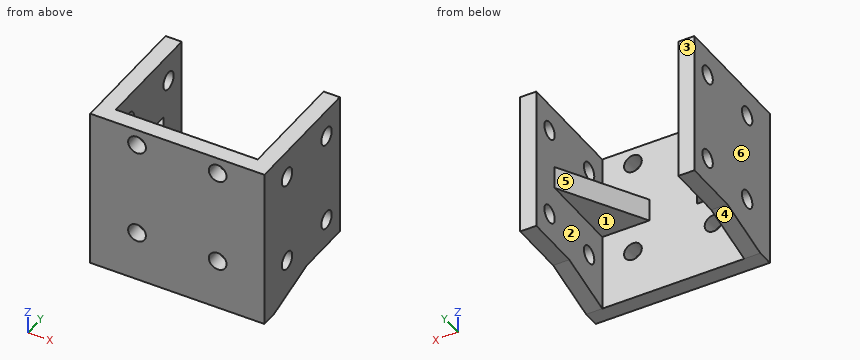
from build123d import *

# Parameters (mm, degrees)
SKETCH1_W               = 54
SKETCH1_H               = 55
BOSS_EXTRUDE1_DEPTH     = 5
SKETCH6_W               = 5
SKETCH6_H               = 45
BOSS_EXTRUDE3_DEPTH     = 35
SKETCH7_R               = 2.75
CUT_EXTRUDE2_DEPTH      = 69.972820734
RIB1_REACH              = 74.61
SKETCH8_WALL_W          = 165.420796688
SKETCH8_WALL_H          = 5
MIRROR2_COPY_1_REACH    = 74.61
MIRROR2_COPY_1_SKETCH_W = 165.420796688
MIRROR2_COPY_1_SKETCH_H = 5
RIB4_REACH              = 57.545
SKETCH9_WALL_W          = 142.246242154
SKETCH9_WALL_H          = 7
SKETCH10_R              = 2.75
CUT_EXTRUDE3_DEPTH      = 53.060061468
SKETCH11_W              = 54
SKETCH11_H              = 5
CUT_EXTRUDE4_DEPTH      = 40


with BuildPart() as part:
    # Sketch1 → Boss-Extrude1 (new body)
    with BuildSketch(Plane(origin=(0, 0, 0), x_dir=(1, 0, 0), z_dir=(0, 1, 0))):
        Rectangle(SKETCH1_W, SKETCH1_H)
    extrude(amount=BOSS_EXTRUDE1_DEPTH)

    # Sketch6 → Boss-Extrude3 (add)
    with BuildSketch(Plane(origin=(0, 5, 0), x_dir=(1, 0, 0), z_dir=(0, 1, 0))):
        with Locations((-24.5, 0)):
            Rectangle(SKETCH6_W, SKETCH6_H)
    boss_extrude3 = extrude(amount=BOSS_EXTRUDE3_DEPTH)

    # Sketch7 → Cut-Extrude2 (cut, through all)
    with BuildSketch(Plane(origin=(-22, 0, 0), x_dir=(0, 0, -1), z_dir=(1, 0, 0))):
        with Locations((-14, 33)):
            Circle(SKETCH7_R)
        with Locations((14, 33)):
            Circle(SKETCH7_R)
        with Locations((14, 12)):
            Circle(SKETCH7_R)
        with Locations((-14, 12)):
            Circle(SKETCH7_R)
    cut_extrude2 = extrude(amount=-CUT_EXTRUDE2_DEPTH, mode=Mode.SUBTRACT)

    # Sketch8 wall → Rib1 (add, up to next)
    with BuildSketch(Plane(origin=(-27, 13.75, -25), x_dir=(0, -0.961523947641, -0.274721127897), z_dir=(0, -0.274721127897, 0.961523947641)), mode=Mode.PRIVATE) as rib1_sk1:
        with Locations((0, 2.5)):
            Rectangle(SKETCH8_WALL_W, SKETCH8_WALL_H)
    rib1_tool1 = extrude(rib1_sk1.sketch, amount=RIB1_REACH, mode=Mode.PRIVATE) - part.part
    rib1 = rib1_tool1.solids().sort_by_distance((-27, 13.75, -25))[0]
    add(rib1)

    # Mirror1: Rib1 across plane
    add(rib1.mirror(Plane.XY))

    # Mirror2: Boss-Extrude3, Cut-Extrude2, Rib1 across plane
    add(boss_extrude3.mirror(Plane(origin=(0, 0, 0), x_dir=(0, 0, 1), z_dir=(1, 0, 0))))
    add(cut_extrude2.mirror(Plane(origin=(0, 0, 0), x_dir=(0, 0, 1), z_dir=(1, 0, 0))), mode=Mode.SUBTRACT)
    add(rib1.mirror(Plane(origin=(0, 0, 0), x_dir=(0, 0, 1), z_dir=(1, 0, 0))))

    # Mirror2 copy 1 sketch → Mirror2 copy 1 (add, up to next)
    with BuildSketch(Plane(origin=(27, 13.75, 25), x_dir=(0, -0.961523947641, 0.274721127897), z_dir=(0, -0.274721127897, -0.961523947641)), mode=Mode.PRIVATE) as mirror2_copy_1_sk1:
        with Locations((0, 2.5)):
            Rectangle(MIRROR2_COPY_1_SKETCH_W, MIRROR2_COPY_1_SKETCH_H)
    mirror2_copy_1_tool1 = extrude(mirror2_copy_1_sk1.sketch, amount=MIRROR2_COPY_1_REACH, mode=Mode.PRIVATE) - part.part
    add(mirror2_copy_1_tool1.solids().sort_by_distance((27, 13.75, 25))[0])

    # Sketch9 wall → Rib4 (add, up to next)
    with BuildSketch(Plane(origin=(-14.710952852, 17.625, 0), x_dir=(0.499999999999, -0.866025403785, 0), z_dir=(0.866025403785, 0.499999999999, 0)), mode=Mode.PRIVATE) as rib4_sk1:
        Rectangle(SKETCH9_WALL_W, SKETCH9_WALL_H)
    rib4_tool1 = extrude(rib4_sk1.sketch, amount=-RIB4_REACH, mode=Mode.PRIVATE) - part.part
    rib4 = rib4_tool1.solids().sort_by_distance((-14.710952852, 17.625, 0))[0]
    add(rib4)

    # Mirror3: Rib4 across plane
    add(rib4.mirror(Plane(origin=(0, 0, 0), x_dir=(0, 0, 1), z_dir=(1, 0, 0))))

    # Sketch10 → Cut-Extrude3 (cut, through all)
    with BuildSketch(Plane(origin=(0, 5, 0), x_dir=(1, 0, 0), z_dir=(0, 1, 0))):
        with Locations(Location((12.5, 11.943211227, 0), (0, 0, 270))):
            Circle(SKETCH10_R)
        with Locations(Location((12.5, -17.5, 0), (0, 0, 270))):
            Circle(SKETCH10_R)
        with Locations(Location((-12.5, -17.5, 0), (0, 0, 270))):
            Circle(SKETCH10_R)
        with Locations(Location((-12.5, 11.943211227, 0), (0, 0, 270))):
            Circle(SKETCH10_R)
    extrude(amount=-CUT_EXTRUDE3_DEPTH, mode=Mode.SUBTRACT)

    # Sketch11 → Cut-Extrude4 (cut)
    with BuildSketch(Plane.XZ):
        with Locations((0, 25)):
            Rectangle(SKETCH11_W, SKETCH11_H)
    extrude(amount=-CUT_EXTRUDE4_DEPTH, mode=Mode.SUBTRACT)


solid = part.part
Can you work these out from the model? Positions are in its coordinate system, mm. Face numbers are marked on the shaded views. A direction names the side the tool comes from. Coordinates: 2 decimals unless noted, no trailing zeros. Order: outer loops, then holes, each group sorted by start corner. A loop starts at its lowest first (then second) coordinate and runs counter-clockwise, first axis right, second up. Notation, with made-up numbers: (-5, 35) - (38, 35) arc R6 ccw to (38, 43) - close; hole circle Ø2 at (-36, -36.75). An arc over 180 degrees is marked (long way). Answer as a JSON object with one key per item and string values. Group by question number.
Q1. I need wall thicknesses on line 1 (Y direction, x = 23.4, z = 14); line 2 (Z direction, x = 25.35, y = 33); line 3 (X direction, y = 2.2, z = 17.5). Which ranges of each line are inside material? Lowest first, please. Write a range as from..to.
Q2. Imagine slicing it at A-A (z = 14). Please give me the cut outline in (x, y).
Q3. Imagine slicing it at C-C (x = 12.5). Please give me the cut outline in (y, z), and give its area (3 significant figures).
Q4. Will these pins go through, and if not, where does the flat tip stop? P1, Ø7, axis at x = 12.5, z = -11.94, coming from the +Y side; P2, Ø7.5, axis at x = -12, y = 13, coming from the -Z side; P3, Ø3.5, axis at y = 33, z = -14, coming from the -X side; P4, Ø11.5, axis at x = -14, y = 11.5, coming from the +Z side.
Q5. We'd pull the mould along X, two halves only. Please class the marked faces 4, 5 and 6: +X half, -X half, draft (parallel to the pull), parting line (faces both ways), or undercut.
Q6. On a 3-axis mill with a long thin cutter (end or side, diameter ignored), from which of +Z, -Z, +X, -X, +Y, -Y can I reach the whole of each face in a straight line? I mean the marked faces 1, 2 and 3. Say none if no direction works.
Q7. Imagine slicing it at B-B (y = 33). Please give me the cut outline in (x, z).
Q8. Imagine slicing it at D-D (y = 3.5). Please give me the cut outline in (x, z), and give its area (3 significant figures).
Determined:
{
 "1": {"line 1": "y = 0..9.25, 14.75..30.25, 35.75..40", "line 2": "z = -22.5..-16.75, -11.25..11.25, 16.75..22.5", "line 3": "x = -27..-15.25, -9.75..9.75, 15.25..27"},
 "2": {"outline": "(-27, 0) - (27, 0) - (27, 9.25) - (22, 9.25) - (22, 5) - (-22, 5) - (-22, 9.25) - (-27, 9.25) - close; (-27, 14.75) - (-22, 14.75) - (-22, 30.25) - (-27, 30.25) - close; (-27, 35.75) - (-22, 35.75) - (-22, 40) - (-27, 40) - close; (22, 14.75) - (27, 14.75) - (27, 30.25) - (22, 30.25) - close; (22, 35.75) - (27, 35.75) - (27, 40) - (22, 40) - close"},
 "3": {"outline": "(0, -27.5) - (5, -27.5) - (5, -14.69) - (0, -14.69) - close; (0, -9.19) - (5, -9.19) - (5, -3.5) - (13.8, -3.5) - (13.8, 3.5) - (5, 3.5) - (5, 14.75) - (0, 14.75) - close; (0, 20.25) - (5, 20.25) - (5, 22.5) - (0, 22.5) - close", "area": "257 mm2"},
 "4": {"P1": "stops at y = 5", "P2": "stops at z = -3.5", "P3": "passes through", "P4": "stops at z = 3.5"},
 "5": {"face 4": "draft", "face 5": "undercut", "face 6": "-X half"},
 "6": {"face 1": "-Z, +Y", "face 2": "+Y", "face 3": "+Z, -Z, +X, -X, +Y"},
 "7": {"outline": "(-27, -22.5) - (-22, -22.5) - (-22, -16.75) - (-27, -16.75) - close; (-27, -11.25) - (-22, -11.25) - (-22, 11.25) - (-27, 11.25) - close; (-27, 16.75) - (-22, 16.75) - (-22, 22.5) - (-27, 22.5) - close; (22, -22.5) - (27, -22.5) - (27, -16.75) - (22, -16.75) - close; (22, -11.25) - (27, -11.25) - (27, 11.25) - (22, 11.25) - close; (22, 16.75) - (27, 16.75) - (27, 22.5) - (22, 22.5) - close"},
 "8": {"outline": "(-27, -27.5) - (27, -27.5) - (27, 22.5) - (-27, 22.5) - close; hole circle Ø5.5 at (-12.5, -11.94); hole circle Ø5.5 at (-12.5, 17.5); hole circle Ø5.5 at (12.5, -11.94); hole circle Ø5.5 at (12.5, 17.5)", "area": "2,600 mm2"}
}
